Can you work these out from the model? Positions are in its coordinate system, mm. Face numbers are marked on the shaded views. A direction names the side the tool comes from. Give positions to 0.01 mm unless a question says otherwise; leave off trailing zeros. Loops run counter-clockwise (first coordinate to the right, second up) from the corner with the lowest first, then second, coordinate; pieces in that order, holes last.
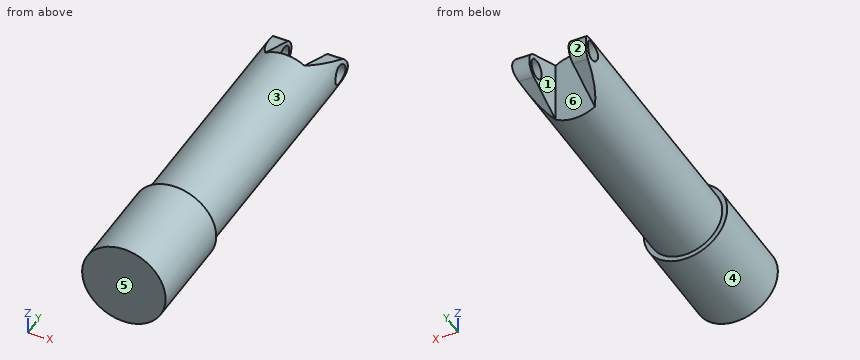
from build123d import *

# Parameters (mm, degrees)
SKETCH_1_R          = 17
EXTRUDE_1_DEPTH     = 40
SKETCH_2_R          = 15
EXTRUDE_2_DEPTH     = 110
SKETCH_3_W          = 16
SKETCH_3_H          = 46
CUT_EXTRUDE_1_DEPTH = 15
SKETCH_4_R          = 4
CUT_EXTRUDE_2_DEPTH = 15
CUT_EXTRUDE_4_DEPTH = 15


with BuildPart() as part:
    # 草图1 → 凸台-拉伸1 (new body)
    with BuildSketch(Plane(origin=(0, 0, 0), x_dir=(1, 0, 0), z_dir=(0, 1, 0))):
        with Locations(Location((0, 0, 0), (0, 0, 270))):
            Circle(SKETCH_1_R)
    extrude(amount=EXTRUDE_1_DEPTH)

    # 草图2 → 凸台-拉伸2 (add)
    with BuildSketch(Plane(origin=(0, 40, 0), x_dir=(1, 0, 0), z_dir=(0, 1, 0))):
        with Locations(Location((0, 0, 0), (0, 0, 270))):
            Circle(SKETCH_2_R)
    extrude(amount=EXTRUDE_2_DEPTH)

    # 草图3 → 切除-拉伸1 (cut, symmetric)
    with BuildSketch(Plane.XY):
        with Locations((0, 150)):
            Rectangle(SKETCH_3_W, SKETCH_3_H)
    extrude(amount=CUT_EXTRUDE_1_DEPTH, both=True, mode=Mode.SUBTRACT)

    # 草图4 → 切除-拉伸2 (cut, symmetric)
    with BuildSketch(Plane(origin=(0, 0, 0), x_dir=(0, 0, -1), z_dir=(1, 0, 0))):
        with Locations(Location((0, 142, 0), (0, 0, 270))):
            Circle(SKETCH_4_R)
    extrude(amount=CUT_EXTRUDE_2_DEPTH, both=True, mode=Mode.SUBTRACT)

    # 草图8 → 切除-拉伸4 (cut, symmetric)
    with BuildSketch(Plane(origin=(0, 0, 0), x_dir=(0, 0, -1), z_dir=(1, 0, 0))):
        with BuildLine():
            Line((-12.68857754, 127), (-5.256345918, 144.263010824))
            ThreePointArc((-5.256345918, 144.263010824), (0, 147.722795681), (5.256345918, 144.263010824))
            Line((5.256345918, 144.263010824), (12.68857754, 127))
            Line((12.68857754, 127), (12.68857754, 150))
            Line((12.68857754, 150), (-12.68857754, 150))
            Line((-12.68857754, 150), (-12.68857754, 127))
        make_face()
    extrude(amount=CUT_EXTRUDE_4_DEPTH, both=True, mode=Mode.SUBTRACT)


solid = part.part
(1) Will these pins go through, and if not, where does the flat tip stop? P1, Ø6.5, axis at y = 142, z = 0, coming from the -X side; P2, Ø3, axis at x = 2, z = 13, coming from the +Y side; P3, Ø6, axis at y = 108.5, z = -3, coming from the -X side; P4, Ø12, axis at y = 93, z = 9, coming from the -X side.
Returned:
P1: passes through
P2: stops at y = 127
P3: stops at x = -15
P4: stops at x = -14.7
(2) Which directions (+Z, -Z, +X, -X, +Y, -Y) give clear straight access to the entire face, cutting with the end or side of a thin tool? Please do the marked faces 1, 2 and 3.
Returned:
face 1: +Z, -Z, +Y
face 2: +X, -X, +Y
face 3: +Y
(3) Thinking about a two-plate mould opening in X: for the marked faces 4, 5 and 6, which applies, pulls with the +X half, pulls with the -X half, needs draft (parallel to the pull), parting line crosses it, or undercut?
Returned:
face 4: parting line crosses it
face 5: needs draft
face 6: undercut
(4) Suppose I cut it at B-B on x = 0. List the corners of the cut face in (y, z) for me.
Returned:
outline: (0, -17) - (40, -17) - (40, -15) - (127, -15) - (127, 15) - (40, 15) - (40, 17) - (0, 17) - close
(5) Please list where these lines run through material, in increasing order: probe 1 along Z at (x, y) = (11.25, 142); probe 2 along Y at (x, z) = (-4, 8); probe 3 along Y at (x, z) = (-10, -13.5).
Returned:
probe 1: z = -6.23 to -4, 4 to 6.23
probe 2: y = 0 to 127
probe 3: y = 0 to 40
(6) Suppose I cut it at A-A on z = 0. List the corners of the cut face in (x, y) for me.
Returned:
outline: (-17, 0) - (17, 0) - (17, 40) - (15, 40) - (15, 138) - (8, 138) - (8, 127) - (-8, 127) - (-8, 138) - (-15, 138) - (-15, 40) - (-17, 40) - close; (-15, 146) - (-8, 146) - (-8, 147.72) - (-15, 147.72) - close; (8, 146) - (15, 146) - (15, 147.72) - (8, 147.72) - close
(7) Suppose I cut it at C-C on y = 142. List the corners of the cut face in (x, z) for me.
Returned:
outline: (-14.46, -4) arc R15 ccw to (-13.64, -6.23) - (-8, -6.23) - (-8, -4) - close; (-14.46, 4) - (-8, 4) - (-8, 6.23) - (-13.64, 6.23) arc R15 ccw to start; (8, -6.23) - (13.64, -6.23) arc R15 ccw to (14.46, -4) - (8, -4) - close; (8, 4) - (14.46, 4) arc R15 ccw to (13.64, 6.23) - (8, 6.23) - close
(8) Suppose I cut it at D-D on x = -11.5. List the corners of the cut face in (y, z) for me, plus the area to 3 significant figures.
Returned:
outline: (0, -12.52) - (40, -12.52) - (40, -9.63) - (134.1, -9.63) - (144.26, -5.26) arc R5.72 ccw to (144.26, 5.26) - (134.1, 9.63) - (40, 9.63) - (40, 12.52) - (0, 12.52) - close; hole circle Ø8 at (142, 0)
area: 2,940 mm2
